Geometry check sheet. Reference: the model listing, model coordinates, mm. A direction names the side the tool comes from. Give positions to 0.01 mm unless a question says otherwise; leave off trailing zeros. Order: outer loops, then holes, each group sorted by start corner. A loop starts at its lowest first (then second) coordinate and runs counter-clockwise, first axis right, second up.
from build123d import *

# Parameters (mm, degrees)
PAD_DEPTH       = 10
SKETCH001_W     = 28.454584
SKETCH001_H     = 18.079305
SKETCH001_W_2   = 14
SKETCH001_H_2   = 12
POCKET_DEPTH    = 1
POCKET001_DEPTH = 2
POCKET002_DEPTH = 5
CHAMFER_SIZE    = 1
CHAMFER001_SIZE = 1
CHAMFER002_SIZE = 1


with BuildPart() as part:
    # Sketch → Pad (new body)
    with BuildSketch(Plane.XY):
        with BuildLine():
            Line((-11.25, 2.35), (-3.8376425055, 2.35))
            ThreePointArc((-2, 4.0311288741), (-3.0374440042, 3.3202310043), (-3.8376425055, 2.35))
            Line((-2, 4.0311288741), (-2, 6))
            Line((-2, 6), (-0.4, 6))
            Line((-0.4, 6), (-0.4, 2.4677925359))
            ThreePointArc((-0.4, 2.4677925359), (0, -2.5), (0.4, 2.4677925359))
            Line((0.4, 6), (0.4, 2.4677925359))
            Line((0.4, 6), (2, 6))
            Line((2, 6), (2, 4.0311288741))
            ThreePointArc((3.8376425055, 2.35), (3.0374440042, 3.3202310043), (2, 4.0311288741))
            Line((3.8376425055, 2.35), (11.25, 2.35))
            Line((11.25, 2.35), (11.25, -2.35))
            Line((11.25, -2.35), (3.8376425055, -2.35))
            ThreePointArc((2, -4.0311288741), (3.0374440042, -3.3202310043), (3.8376425055, -2.35))
            Line((2, -4.0311288741), (2, -6))
            Line((2, -6), (-2, -6))
            Line((-2, -6), (-2, -4.0311288741))
            ThreePointArc((-3.8376425055, -2.35), (-3.0374440042, -3.3202310043), (-2, -4.0311288741))
            Line((-3.8376425055, -2.35), (-11.25, -2.35))
            Line((-11.25, -2.35), (-11.25, 2.35))
        make_face()
    extrude(amount=PAD_DEPTH)

    # Sketch001 (on Face21 of Pad) → Pocket (cut)
    with BuildSketch(Plane(origin=(0, 0, 0), x_dir=(1, 0, 0), z_dir=(0, 0, -1))):
        with Locations((-1.003043, -0.4011775)):
            Rectangle(SKETCH001_W, SKETCH001_H)
        Rectangle(SKETCH001_W_2, SKETCH001_H_2, mode=Mode.SUBTRACT)
    extrude(amount=-POCKET_DEPTH, mode=Mode.SUBTRACT)

    # Sketch002 (on Face6 of Pocket) → Pocket001 (cut)
    with BuildSketch(Plane.XY.offset(10)):
        with BuildLine():
            ThreePointArc((-2, 4.0311288741), (-4.5, 0), (-2, -4.0311288741))
            Line((-2, -4.0311288741), (-2, -6))
            Line((-2, -6), (2, -6))
            Line((2, -6), (2, -4.0311288741))
            ThreePointArc((2, -4.0311288741), (4.5, 0), (2, 4.0311288741))
            Line((2, 6), (2, 4.0311288741))
            Line((-2, 6), (2, 6))
            Line((-2, 4.0311288741), (-2, 6))
        make_face()
    extrude(amount=-POCKET001_DEPTH, mode=Mode.SUBTRACT)

    # Sketch003 (on Face1 of Pocket001) → Pocket002 (cut)
    with BuildSketch(Plane.XZ.offset(2.35)):
        Polygon((-9.05, 10), (-9.05, 8.5), (-10.25, 8.5), (-10.25, 3), (-7.0376425055, 3), (-7.0376425055, 10), align=None)
        Polygon((9.05, 10), (9.05, 8.5), (10.25, 8.5), (10.25, 3), (7.0376425055, 3), (7.0376425055, 10), align=None)
    extrude(amount=-POCKET002_DEPTH, mode=Mode.SUBTRACT)

    # Chamfer
    chamfer_edges = [part.edges().sort_by_distance(p)[0] for p in [
        (0, -2.5, 0),
    ]]
    chamfer(chamfer_edges, length=CHAMFER_SIZE)

    # Chamfer001
    chamfer001_edges = [part.edges().sort_by_distance(p)[0] for p in [
        (-7.037643, 0, 10),
        (7.037643, 0, 10),
    ]]
    chamfer(chamfer001_edges, length=CHAMFER001_SIZE)

    # Chamfer002
    chamfer002_edges = [part.edges().sort_by_distance(p)[0] for p in [
        (-9.05, 0, 10),
        (9.05, 0, 10),
    ]]
    chamfer(chamfer002_edges, length=CHAMFER002_SIZE)


solid = part.part
Item 1: Set-up check for faces 5 (the flat face through (7.038, 0, 6)), 6 (the flat face through (0, -3, 8)), 7 (the flat face through (-2, -5, 4)), 8 (the flat face through (-6.8, 2.35, 4.9)): record each of +Z, -Z, +X, -X, +Y, -Y from which the full face is reachable in a straight line by a thin tool's end or side.
Reported:
face 5: +Z, +Y, -Y
face 6: +Z
face 7: +Z, -Z, -X, -Y
face 8: +Z, -Z, -X, +Y
Item 2: Draft check along Z on faces 1 (the flat face through (-2, -3.1, 0)), 2 (the flat face through (10.25, 0, 6)), 3 (the flat face through (9, 0, 3)), 4 (the flat face through (-7.038, 0, 6)). Enter one of: released by +Z, released by -Z, zero draft, split by the parting line, or undercut.
Reported:
face 1: released by -Z
face 2: undercut
face 3: undercut
face 4: zero draft
Item 3: Scan lines: L1, parallel to X at y = 0, z = 3.75; L2, parallel to X at y = 5.5, z = 6.5; L3, parallel to X at y = 0.75, z = 6.25. Record each from-to range of solid material in increasing order.
Reported:
L1: x = -11.25 to -10.25, -7.04 to -2.5, 2.5 to 7.04, 10.25 to 11.25
L2: x = -2 to -0.4, 0.4 to 2
L3: x = -11.25 to -10.25, -7.04 to -2.38, 2.38 to 7.04, 10.25 to 11.25
Item 4: Sectioned sample at C-C (x = 0). Enter the section's corners in (y, z).
Reported:
outline: (-6, 0) - (-3.5, 0) - (-2.5, 1) - (-2.5, 8) - (-6, 8) - close
Item 5: Sectioned sample at B-B (z = 7.25). Enter the section's corners in (x, y).
Reported:
outline: (-11.25, -2.35) - (-10.25, -2.35) - (-10.25, 2.35) - (-11.25, 2.35) - close; (-7.04, -2.35) - (-3.84, -2.35) arc R4.5 ccw to (-2, -4.03) - (-2, -6) - (2, -6) - (2, -4.03) arc R4.5 ccw to (3.84, -2.35) - (7.04, -2.35) - (7.04, 2.35) - (3.84, 2.35) arc R4.5 ccw to (2, 4.03) - (2, 6) - (0.4, 6) - (0.4, 2.47) arc R2.5 cw (long way) to (-0.4, 2.47) - (-0.4, 6) - (-2, 6) - (-2, 4.03) arc R4.5 ccw to (-3.84, 2.35) - (-7.04, 2.35) - close; (10.25, -2.35) - (11.25, -2.35) - (11.25, 2.35) - (10.25, 2.35) - close
Item 6: Gauge pin test, flat ends, axial feed: pin 1 (6 mm diameter, centred on x = 5.5, z = 4.5, fed in from -Y); pin 2 (3 mm diameter, centred on y = 4.5, z = 4, fed in from +X); pin 3 (0.6 mm diameter, centred on x = 10, y = -0.5, fed in from -Z). Record the tip position at first contact, or that the pin passes through.
Reported:
pin 1: stops at y = -3.74
pin 2: stops at x = 3.35
pin 3: stops at z = 1
Item 7: Sectioned sample at D-D (z = 0.75). Enter the section's corners in (x, y).
Reported:
outline: (-7, -2.35) - (-3.84, -2.35) arc R4.5 ccw to (-2, -4.03) - (-2, -6) - (2, -6) - (2, -4.03) arc R4.5 ccw to (3.84, -2.35) - (7, -2.35) - (7, 2.35) - (3.84, 2.35) arc R4.5 ccw to (2, 4.03) - (2, 6) - (0.4, 6) - (0.4, 2.72) arc R2.75 cw (long way) to (-0.4, 2.72) - (-0.4, 6) - (-2, 6) - (-2, 4.03) arc R4.5 ccw to (-3.84, 2.35) - (-7, 2.35) - close
